Build history of the part. All positions in model axes, mm. Round coordinates to 2 decimals unless told otherwise and drop trailing zeros. Answer in a Markdown table with one row per item.
Autodesk Inventor part; units mm, degrees
ref_plane "YZ Plane" through (0, 0, 0) normal (1, 0, 0) x (0, 1, 0)
ref_plane "XZ Plane" through (0, 0, 0) normal (0, 1, 0) x (-1, 0, 0)
ref_plane "XY Plane" through (0, 0, 0) normal (0, 0, 1) x (1, 0, 0)
sketch "Sketch1" plane through (0, 0, 0) normal (0, 1, 0) x (-1, 0, 0)
  line L0 (6.35, 0) -> (1365.25, 0)
  line L1 (1371.6, -6.35) -> (1371.6, -1365.25)
  line L2 (1365.25, -1371.6) -> (6.35, -1371.6)
  line L3 (0, -1365.25) -> (0, -6.35)
  line L4 (1346.2, -1346.2) -> (1346.2, -25.4)
  line L5 (1346.2, -25.4) -> (25.4, -25.4)
  line L6 (25.4, -25.4) -> (25.4, -1346.2)
  line L7 (25.4, -1346.2) -> (1346.2, -1346.2)
  line L8 (1320.8, -50.8) -> (1320.8, -1320.8)
  line L9 (1320.8, -1320.8) -> (50.8, -1320.8)
  line L10 (50.8, -1320.8) -> (50.8, -50.8)
  line L11 (50.8, -50.8) -> (1320.8, -50.8)
  line L12 (1320.8, -50.8) -> (1346.2, -25.4)
  line L13 (1320.8, -1320.8) -> (1346.2, -1346.2)
  line L14 (50.8, -1320.8) -> (25.4, -1346.2)
  line L15 (50.8, -50.8) -> (25.4, -25.4)
  line L16 (1219.2, -482.6) -> (1016, -482.6)
  line L17 (1016, -482.6) -> (1016, -889)
  line L18 (1016, -889) -> (1219.2, -889)
  line L19 (1219.2, -889) -> (1219.2, -482.6)
  line L20 (355.6, -482.6) -> (152.4, -482.6)
  line L21 (152.4, -482.6) -> (152.4, -889)
  line L22 (152.4, -889) -> (355.6, -889)
  line L23 (355.6, -889) -> (355.6, -482.6)
  line L24 (889, -1016) -> (482.6, -1016)
  line L25 (482.6, -1016) -> (482.6, -1219.2)
  line L26 (482.6, -1219.2) -> (889, -1219.2)
  line L27 (889, -1219.2) -> (889, -1016)
  line L28 (889, -152.4) -> (482.6, -152.4)
  line L29 (482.6, -152.4) -> (482.6, -355.6)
  line L30 (482.6, -355.6) -> (889, -355.6)
  line L31 (889, -355.6) -> (889, -152.4)
  circle A0 centre (685.8, -685.8) radius 254
  line L32 (889, -127) -> (482.6, -127)
  line L33 (457.2, -127) -> (457.2, -381)
  line L34 (457.2, -381) -> (914.4, -381)
  line L35 (914.4, -381) -> (914.4, -127)
  line L36 (1244.6, -457.2) -> (990.6, -457.2)
  line L37 (990.6, -457.2) -> (990.6, -914.4)
  line L38 (990.6, -914.4) -> (1244.6, -914.4)
  line L39 (1244.6, -889) -> (1244.6, -482.6)
  line L40 (914.4, -990.6) -> (457.2, -990.6)
  line L41 (457.2, -990.6) -> (457.2, -1244.6)
  line L42 (482.6, -1244.6) -> (889, -1244.6)
  line L43 (914.4, -1244.6) -> (914.4, -990.6)
  line L44 (381, -457.2) -> (127, -457.2)
  line L45 (127, -482.6) -> (127, -889)
  line L46 (127, -914.4) -> (381, -914.4)
  line L47 (381, -914.4) -> (381, -457.2)
  line L48 (152.4, -482.6) -> (50.8, -482.6)
  line L49 (127, -457.2) -> (50.8, -457.2)
  line L50 (152.4, -889) -> (50.8, -889)
  line L51 (127, -914.4) -> (50.8, -914.4)
  line L52 (355.6, -889) -> (381, -889)
  line L53 (355.6, -482.6) -> (381, -482.6)
  line L54 (457.2, -1244.6) -> (457.2, -1320.8)
  line L55 (482.6, -1219.2) -> (482.6, -1320.8)
  line L56 (889, -1219.2) -> (889, -1320.8)
  line L57 (914.4, -1244.6) -> (914.4, -1320.8)
  line L58 (1244.6, -914.4) -> (1320.8, -914.4)
  line L59 (1219.2, -889) -> (1320.8, -889)
  line L60 (1219.2, -482.6) -> (1320.8, -482.6)
  line L61 (1244.6, -457.2) -> (1320.8, -457.2)
  line L62 (889, -152.4) -> (889, -50.8)
  line L63 (914.4, -127) -> (914.4, -50.8)
  line L64 (482.6, -152.4) -> (482.6, -50.8)
  line L65 (457.2, -127) -> (457.2, -50.8)
  line L66 (889, -1016) -> (889, -990.6)
  line L67 (482.6, -1016) -> (482.6, -990.6)
  line L68 (1016, -889) -> (990.6, -889)
  line L69 (1016, -482.6) -> (990.6, -482.6)
  line L70 (889, -355.6) -> (889, -381)
  line L71 (482.6, -355.6) -> (482.6, -381)
  line L72 (914.4, -381) -> (990.6, -457.2)
  line L73 (990.6, -482.6) -> (889, -381)
  line L74 (990.6, -914.4) -> (914.4, -990.6)
  line L75 (889, -990.6) -> (990.6, -889)
  line L76 (381, -914.4) -> (457.2, -990.6)
  line L77 (482.6, -990.6) -> (381, -889)
  line L78 (457.2, -381) -> (381, -457.2)
  line L79 (482.6, -381) -> (381, -482.6)
  line L80 (1257.3, -50.8) -> (1320.8, -114.3)
  line L81 (1320.8, -1257.3) -> (1257.3, -1320.8)
  line L82 (50.8, -1257.3) -> (114.3, -1320.8)
  line L83 (50.8, -114.3) -> (114.3, -50.8)
  line L84 (68.7605, -132.2605) -> (132.2605, -68.7605)
  line L85 (68.7605, -1239.3395) -> (132.2605, -1302.8395)
  line L86 (1302.8395, -1239.3395) -> (1239.3395, -1302.8395)
  line L87 (1239.3395, -68.7605) -> (1302.8395, -132.2605)
  line L88 (1302.8395, -132.2605) -> (1320.8, -150.221)
  line L89 (1239.3395, -68.7605) -> (1221.379, -50.8)
  line L90 (1302.8395, -1239.3395) -> (1320.8, -1221.379)
  line L91 (1239.3395, -1302.8395) -> (1221.379, -1320.8)
  line L92 (132.2605, -1302.8395) -> (150.221, -1320.8)
  line L93 (68.7605, -1239.3395) -> (50.8, -1221.379)
  line L94 (132.2605, -68.7605) -> (150.221, -50.8)
  line L95 (68.7605, -132.2605) -> (50.8, -150.221)
  line L96 (1365.25, 0) -> (1371.6, -6.35)
  line L97 (1371.6, -1365.25) -> (1365.25, -1371.6)
  line L98 (6.35, -1371.6) -> (0, -1365.25)
  line L99 (6.35, 0) -> (0, -6.35)
  point P0 (0, 0)
  point P1 (1371.6, -1371.6)
  point P2 (1371.6, 0)
  point P3 (0, -1371.6)
  dimension "d0" = 1371.6
  dimension "d1" = 1371.6
  dimension "d2" = 25.4
  dimension "d3" = 25.4
  dimension "d4" = 203.2
  dimension "d5" = 406.4
  dimension "d6" = 203.2
  dimension "d7" = 406.4
  dimension "d8" = 406.4
  dimension "d9" = 203.2
  dimension "d10" = 406.4
  dimension "d11" = 203.2
  dimension "d12" = 101.6
  dimension "d13" = 101.6
  dimension "d14" = 101.6
  dimension "d15" = 101.6
  dimension "d16" = 431.8
  dimension "d17" = 431.8
  dimension "d18" = 431.8
  dimension "d19" = 431.8
  dimension "d20" = 508
  dimension "d21" = 25.4
  dimension "d22" = 25.4
  dimension "d23" = 25.4
  dimension "d24" = 25.4
  dimension "d25" = 45
  dimension "d26" = 63.5
  dimension "d27" = 45
  dimension "d28" = 45
  dimension "d29" = 45
  dimension "d30" = 25.4
  dimension "d31" = 25.4
  dimension "d32" = 25.4
  dimension "d33" = 25.4
  dimension "d34" = 6.35
  dimension "d35" = 6.35
  dimension "d36" = 6.35
  dimension "d37" = 6.35
  dimension "d38" = 6.35
  dimension "d39" = 6.35
  dimension "d40" = 6.35
  dimension "d41" = 6.35
extrude "Extrusion1" add sketch "Sketch1" along normal blind 76.2 contours L13 L8 L12 L4
sketch "Sketch2" plane through (-1320.8, 0, -50.8) normal (0.7071, 0, 0.7071) x (0.7071, 0, -0.7071)
  point P0 (898.0256, 0)
sketch "Sketch3" plane through (-1320.8, 0, -50.8) normal (0.7071, 0, 0.7071) x (0.7071, 0, -0.7071)
  circle A0 centre (-17.9578, 63.5) radius 1.5875
  circle A1 centre (-17.9578, 12.7) radius 1.5875
  line L0 (0, 0) -> (0, 76.2)
  line L1 (-35.921, 76.2) -> (0, 76.2)
  line L2 (-35.921, 0) -> (0, 0)
  point P0 (898.0256, 0)
  dimension "d44" = 3.175
  dimension "d45" = 3.175
  dimension "d46" = 17.9578
  dimension "d47" = 17.9578
  dimension "d48" = 12.7
  dimension "d49" = 12.7
extrude "Extrusion2" cut sketch "Sketch3" against normal blind 76.2
sketch "Sketch4" plane through (-1346.2, 0, -1346.2) normal (0.7071, 0, -0.7071) x (-0.7071, 0, -0.7071)
  circle A0 centre (-17.9632, 63.5) radius 1.5875
  circle A1 centre (-17.9632, 12.7) radius 1.5875
  line L0 (-35.921, 0) -> (-35.921, 76.2)
  line L1 (-35.921, 0) -> (0, 0)
  line L2 (-35.921, 76.2) -> (0, 76.2)
  point P0 (-1903.8143, 0)
  dimension "d52" = 3.175
  dimension "d53" = 3.175
  dimension "d54" = 17.9578
  dimension "d55" = 17.9578
  dimension "d56" = 12.7
  dimension "d57" = 12.7
extrude "Extrusion3" cut sketch "Sketch4" against normal blind 76.2
hole "Hole1" at (-1346.2, 12.7, -50.8038) direction (-0.7071, 0, -0.7071) diameter 6.35 depth 3.81
hole "Hole2" at (-1346.2, 63.5, -50.8038) direction (-0.7071, 0, -0.7071) diameter 6.35 depth 3.81
hole "Hole3" at (-1346.2, 63.5, -1320.7962) direction (-0.7071, 0, 0.7071) diameter 6.35 depth 3.81
hole "Hole4" at (-1346.2, 12.7, -1320.7962) direction (-0.7071, 0, 0.7071) diameter 6.35 depth 3.81
hole "Hole5" at (-1346.2, 12.7, -1320.7962) direction (0.7071, 0, -0.7071) diameter 6.35 depth 3.81
hole "Hole6" at (-1346.2, 63.5, -1320.7962) direction (0.7071, 0, -0.7071) diameter 6.35 depth 3.81
hole "Hole7" at (-1346.2, 12.7, -50.8038) direction (0.7071, 0, 0.7071) diameter 6.35 depth 3.81
hole "Hole8" at (-1346.2, 63.5, -50.8038) direction (0.7071, 0, 0.7071) diameter 6.35 depth 3.81
sketch "Sketch5" plane through (-1320.8, 0, -50.8) normal (1, 0, 0) x (0, 0, -1)
  line L0 (406.4, 0) -> (406.4, 76.2)
  line L1 (0, 76.2) -> (1270, 76.2)
  line L2 (431.8, 0) -> (431.8, 76.2)
  line L3 (431.8, 76.2) -> (406.4, 76.2)
  circle A0 centre (419.1, 63.5) radius 1.5875
  circle A1 centre (419.1, 12.7) radius 1.5875
  line L4 (0, 0) -> (1270, 0)
  line L5 (838.2, 0) -> (838.2, 76.2)
  line L6 (863.6, 0) -> (863.6, 76.2)
  line L7 (838.2, 76.2) -> (863.6, 76.2)
  circle A2 centre (850.9, 63.5) radius 1.5875
  circle A3 centre (850.9, 12.7) radius 1.5875
  point P0 (-50.8, 0)
  point P1 (431.8, 0)
  dimension "d132" = 3.175
  dimension "d133" = 3.175
  dimension "d134" = 12.7
  dimension "d135" = 12.7
  dimension "d136" = 12.7
  dimension "d137" = 12.7
  dimension "d138" = 3.175
  dimension "d139" = 3.175
  dimension "d140" = 12.7
  dimension "d141" = 12.7
  dimension "d142" = 12.7
  dimension "d143" = 12.7
extrude "Extrusion4" cut sketch "Sketch5" against normal blind 76.2 contours A0 | A1 | A2 | A3
chamfer "Chamfer1" distance 3.175 angle 45 4 edges at (-1346.2, 12.7, -468.3125) (-1346.2, 63.5, -468.3125) (-1346.2, 12.7, -900.1125) (-1346.2, 63.5, -900.1125)
sketch "Sketch6" plane through (-1320.8, 0, -50.8) normal (1, 0, 0) x (0, 0, -1)
  circle A0 centre (35.9156, 63.5) radius 1.5875
  circle A1 centre (59.1312, 63.5) radius 1.5875
  circle A2 centre (35.9156, 38.1) radius 1.5875
  circle A3 centre (59.1312, 38.1) radius 1.5875
  circle A4 centre (35.9156, 12.7) radius 1.5875
  circle A5 centre (59.1312, 12.7) radius 1.5875
  line L0 (0, 76.2) -> (1270, 76.2)
  line L1 (0, 0) -> (1270, 0)
  line L2 (0, 0) -> (0, 76.2)
  line L3 (635, 354.9927) -> (635, -254.0092)
  line L4 (-25.4, 0) -> (-25.4, 76.2)
  circle A6 centre (1234.0844, 63.5) radius 1.5875
  circle A7 centre (1210.8688, 63.5) radius 1.5875
  circle A8 centre (1234.0844, 38.1) radius 1.5875
  circle A9 centre (1210.8688, 38.1) radius 1.5875
  circle A10 centre (1234.0844, 12.7) radius 1.5875
  circle A11 centre (1210.8688, 12.7) radius 1.5875
  line L5 (1270, 0) -> (1270, 76.2)
  line L6 (1295.4, 0) -> (1295.4, 76.2)
  point P0 (-50.8, 0)
  point P1 (1320.8, 0)
  dimension "d149" = 3.175
  dimension "d150" = 3.175
  dimension "d151" = 3.175
  dimension "d152" = 3.175
  dimension "d153" = 3.175
  dimension "d154" = 3.175
  dimension "d155" = 12.7
  dimension "d156" = 12.7
  dimension "d157" = 38.1
  dimension "d158" = 38.1
  dimension "d159" = 12.7
  dimension "d160" = 12.7
  dimension "d161" = 35.9156
  dimension "d162" = 35.9156
  dimension "d163" = 35.9156
  dimension "d164" = 23.2156
  dimension "d165" = 23.2156
  dimension "d166" = 23.2156
  dimension "d172" = 660.4
extrude "Extrusion5" cut sketch "Sketch6" against normal blind 76.2 contours A0 | A1 | A2 | A3 | A4 | A5 | A6 | A7 | A8 | A9 | A10 | A11
chamfer "Chamfer2" distance 3.175 angle 45 12 edges at (-1346.2, 12.7, -85.1281) (-1346.2, 12.7, -108.3437) (-1346.2, 38.1, -85.1281) (-1346.2, 63.5, -85.1281) (-1346.2, 38.1, -108.3437) (-1346.2, 63.5, -108.3437) (-1346.2, 63.5, -1283.2969) (-1346.2, 63.5, -1260.0813) (-1346.2, 38.1, -1283.2969) (-1346.2, 38.1, -1260.0813) (-1346.2, 12.7, -1283.2969) (-1346.2, 12.7, -1260.0813)
properties part number "Main frame Piece X4"
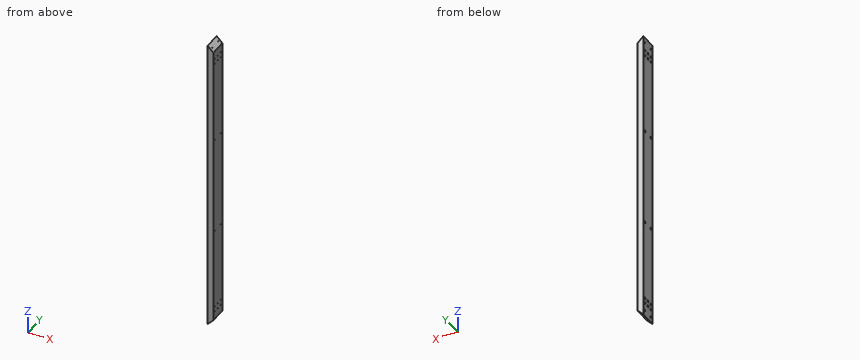
Q1. Saw through at A-A on x = -1325. State how many separate pieces and enclosed holes the cut face has, plus the area to 3 significant figures.
A:
| item | result |
|---|---|
| separate pieces | 1 |
| enclosed holes | 16 |
| area | 97,300 mm² |
Q2. Drop flat-ended pins along their axis: P1, Ø3, axis at y = 12.7, z = -469.9, coming from the -X side; P2, Ø5, axis at x = -1341, y = 66.5, coming from the +Z side; P3, Ø10, axis at x = -1340.5, y = 27.5, coming from the -Z side; P4, Ø4, axis at y = 12.7, z = -1284.88, coming from the -X side. Give the stop position or say it passes through.
A:
| item | result |
|---|---|
| P1 | through |
| P2 | z = -28.1 |
| P3 | z = -1345.5 |
| P4 | x = -1343.44 |
Q3. Wall check: line 1 (Y direction, x = -1332.75, z = -901.7); line 2 (X direction, y = 17, z = -1261.5); line 3 (Z direction, x = -1337.5, y = 39.5). Give the ranges that are in metal, low to high. Write a range as [from, to].
A:
| item | result |
|---|---|
| line 1 | [0, 11.11], [14.29, 61.91], [65.09, 76.2] |
| line 2 | [-1345.74, -1320.8] |
| line 3 | [-1337.5, -1285.63], [-1284.14, -1262.42], [-1260.92, -110.68], [-109.18, -87.46], [-85.97, -34.1] |
